```python
from build123d import *

# Parameters (mm, degrees)
SKETCH1_W           = 20
SKETCH1_H           = 20
BOSS_EXTRUDE1_DEPTH = 22
SKETCH2_W           = 12
SKETCH2_H           = 14
CUT_EXTRUDE1_DEPTH  = 16
SKETCH3_W           = 22
SKETCH3_H           = 5
BOSS_EXTRUDE2_DEPTH = 2
LPATTERN1_COUNT     = 6
LPATTERN1_PITCH     = 22
SKETCH4_W           = 22
SKETCH4_H           = 15
BOSS_EXTRUDE3_DEPTH = 2
SKETCH5_W           = 22
SKETCH5_H           = 20
BOSS_EXTRUDE4_DEPTH = 2
SKETCH6_W           = 122
SKETCH6_H           = 2
CUT_EXTRUDE2_DEPTH  = 2
SKETCH7_W           = 134
SKETCH7_H           = 22
BOSS_EXTRUDE5_DEPTH = 6


with BuildPart() as part:
    # Sketch1 → Boss-Extrude1 (new body)
    with BuildSketch(Plane.XY):
        with Locations((10, 10)):
            Rectangle(SKETCH1_W, SKETCH1_H)
    extrude(amount=BOSS_EXTRUDE1_DEPTH)

    # Sketch2 → Cut-Extrude1 (cut)
    with BuildSketch(Plane.XZ):
        with Locations((10, 11)):
            Rectangle(SKETCH2_W, SKETCH2_H)
    extrude(amount=-CUT_EXTRUDE1_DEPTH, mode=Mode.SUBTRACT)

    # Sketch3 → Boss-Extrude2 (add)
    with BuildSketch(Plane(origin=(20, 0, 0), x_dir=(0, 0, -1), z_dir=(1, 0, 0))):
        with Locations((-11, 2.5)):
            Rectangle(SKETCH3_W, SKETCH3_H)
    extrude(amount=BOSS_EXTRUDE2_DEPTH)


with BuildPart() as lpattern1_1:
    # LPattern1: pattern copy
    add(part.part.moved(Location(Vector(1, 0, 0) * (1 * LPATTERN1_PITCH))))


with BuildPart() as lpattern1_2:
    # LPattern1: pattern copy
    add(part.part.moved(Location(Vector(1, 0, 0) * (2 * LPATTERN1_PITCH))))


with BuildPart() as lpattern1_3:
    # LPattern1: pattern copy
    add(part.part.moved(Location(Vector(1, 0, 0) * (3 * LPATTERN1_PITCH))))


with BuildPart() as lpattern1_4:
    # LPattern1: pattern copy
    add(part.part.moved(Location(Vector(1, 0, 0) * (4 * LPATTERN1_PITCH))))


with BuildPart() as lpattern1_5:
    # LPattern1: pattern copy
    add(part.part.moved(Location(Vector(1, 0, 0) * (5 * LPATTERN1_PITCH))))


with BuildPart() as part_1:
    add(part.part)

    # Combine1: union LPattern1_1, LPattern1_2, LPattern1_3, LPattern1_4, LPattern1_5
    add(lpattern1_1.part)
    add(lpattern1_2.part)
    add(lpattern1_3.part)
    add(lpattern1_4.part)
    add(lpattern1_5.part)

    # Sketch4 → Boss-Extrude3 (add)
    with BuildSketch(Plane(origin=(130, 0, 0), x_dir=(0, 0, -1), z_dir=(1, 0, 0))):
        with Locations((-11, 12.5)):
            Rectangle(SKETCH4_W, SKETCH4_H)
    extrude(amount=BOSS_EXTRUDE3_DEPTH)

    # Sketch5 → Boss-Extrude4 (add)
    with BuildSketch(Plane.ZY):
        with Locations((11, 10)):
            Rectangle(SKETCH5_W, SKETCH5_H)
    extrude(amount=BOSS_EXTRUDE4_DEPTH)

    # Sketch6 → Cut-Extrude2 (cut)
    with BuildSketch(Plane(origin=(0, 0, 0), x_dir=(-1, 0, 0), z_dir=(0, -1, 0))):
        with Locations((-65, -11)):
            Rectangle(SKETCH6_W, SKETCH6_H)
    extrude(amount=-CUT_EXTRUDE2_DEPTH, mode=Mode.SUBTRACT)

    # Sketch7 → Boss-Extrude5 (add)
    with BuildSketch(Plane.XZ):
        with Locations((65, 11)):
            Rectangle(SKETCH7_W, SKETCH7_H)
    extrude(amount=BOSS_EXTRUDE5_DEPTH)


solid = part_1.part
```
Source: CAD feature listing. Evaluate the final solid. Frame: model axes, mm. A direction names the side the tool comes from. Give positions to 0.01 mm unless a question says otherwise; leave off trailing zeros. Order: outer loops, then holes, each group sorted by start corner. A loop starts at its lowest first (then second) coordinate and runs counter-clockwise, first axis right, second up.
(1) Section query A-A (y = 17.25). Return the cut outline in (x, z), plus the area to 3 significant figures.
(2) Section query B-B (x = 49.5). Return the cut outline in (y, z), plus the area to 3 significant figures.
(3) Pull-direction query (Y, two-part tool) for faces 4 (the face through (64, 4, 22)), 5 (the face through (9, 20, 11)), 6 (the face through (48, 8, 11)), 7 (the face through (4, 8, 11)); classes: +Y half, -Y half, draft (parallel to the pull), parting line (faces both ways), or undercut.
(4) Contact query for a flat-ended pin moving along its axis: P1, Ø1.6, axis at x = 43, z = 10, coming from the +Y side. Output: stop coordinate, or through.
(5) Section query D-D (z = 2.75). Return the cut outline in (x, y).
(6) Material intervals for line 1 along X through (y, z) = (7, 19.5); line 2 along Y through (x, z) = (100.5, 14.5); line 3 along Z through (x, y) = (119.5, 12), sorted ascending.
(7) Section query C-C (y = 8.75). State how many separate pieces and enclosed holes the cut face has, plus the area to 3 significant figures.
(8) Access query for faces 1 (the face through (54, 16, 11)), 2 (the face through (22, 12, 11)), 3 (the face through (98, 20, 11)). Directions: +Z, -Z, +X, -X, +Y, -Y. A direction counts if a zero-diameter tool reaches every point of the face in a straight line with its end or side. Return the directions, or none.
Outcome:
1. outline: (-2, 0) - (20, 0) - (20, 22) - (-2, 22) - close; (22, 0) - (42, 0) - (42, 22) - (22, 22) - close; (44, 0) - (64, 0) - (64, 22) - (44, 22) - close; (66, 0) - (86, 0) - (86, 22) - (66, 22) - close; (88, 0) - (108, 0) - (108, 22) - (88, 22) - close; (110, 0) - (132, 0) - (132, 22) - (110, 22) - close
1. area: 2,730 mm2
2. outline: (-6, 0) - (20, 0) - (20, 22) - (-6, 22) - close; hole (0, 4) - (16, 4) - (16, 18) - (0, 18) - close
2. area: 348 mm2
3. face 4: draft
3. face 5: +Y half
3. face 6: undercut
3. face 7: undercut
4. P1: stops at y = 5
5. outline: (-2, -6) - (132, -6) - (132, 20) - (110, 20) - (110, 5) - (108, 5) - (108, 20) - (88, 20) - (88, 5) - (86, 5) - (86, 20) - (66, 20) - (66, 5) - (64, 5) - (64, 20) - (44, 20) - (44, 5) - (42, 5) - (42, 20) - (22, 20) - (22, 5) - (20, 5) - (20, 20) - (-2, 20) - close
6. line 1: x = -2 to 20, 22 to 42, 44 to 64, 66 to 86, 88 to 108, 110 to 132
6. line 2: y = -6 to 0, 16 to 20
6. line 3: z = 0 to 4, 18 to 22
7. separate pieces: 6
7. enclosed holes: 6
7. area: 1,720 mm2
8. face 1: none
8. face 2: +Z, -Z, +Y
8. face 3: +Z, -Z, +X, -X, +Y
